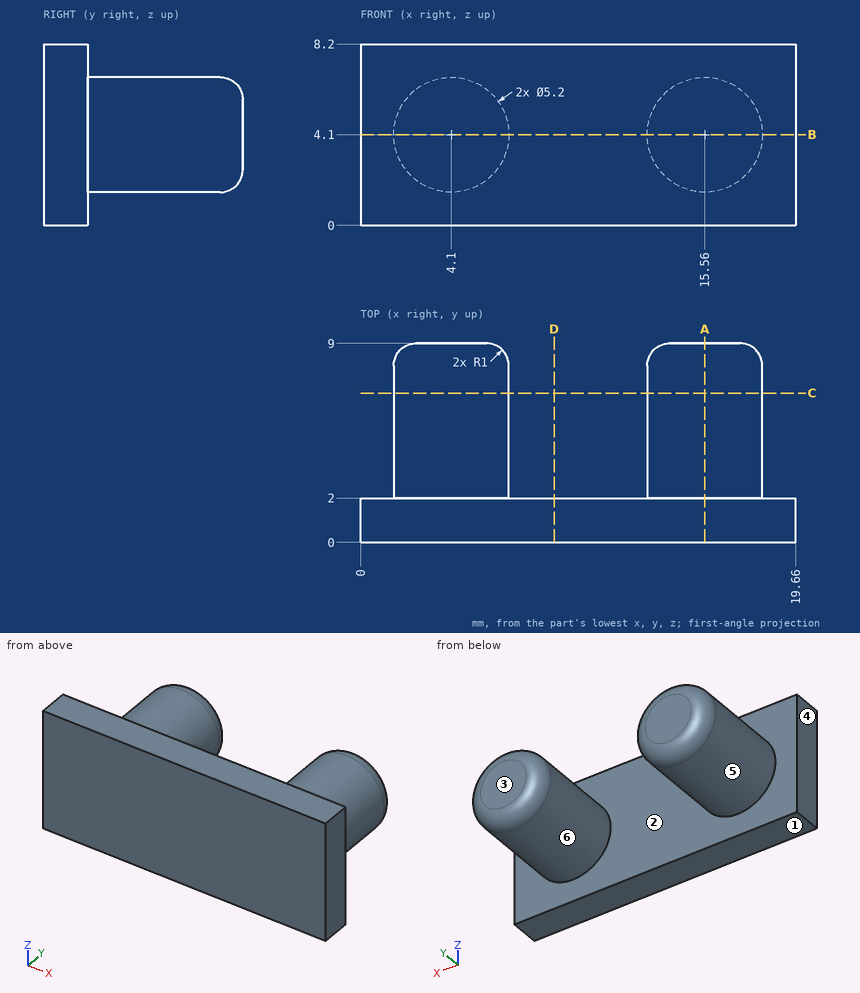
Can you work these out from the drawing? Everything is in mm from the part's minimum corner. A direction names the side the tool comes from. Round coordinates to 2 decimals unless told otherwise and drop trailing zeros. Loops run counter-clockwise (first coordinate to the right, second up) from the corner with the lowest first, then second, coordinate; pieces in that order, holes last. Notation, with made-up numbers: (-36.5, -1.75) -> (-7.5, -1.75) arc R20 cw to (-7.5, 7.25) -> close; hole circle Ø9 at (28, -1). An arc over 180 degrees is marked (long way). Put each result on its own line as item: value.
Q1. I want a section at B-B on z = 4.1. Write out the boundary of the cut face in (x, y), and give its area (3 significant figures).
Checks:
outline: (0, 0) -> (19.66, 0) -> (19.66, 2) -> (18.16, 2) -> (18.16, 8) arc R1 ccw to (17.16, 9) -> (13.96, 9) arc R1 ccw to (12.96, 8) -> (12.96, 2) -> (6.7, 2) -> (6.7, 8) arc R1 ccw to (5.7, 9) -> (2.5, 9) arc R1 ccw to (1.5, 8) -> (1.5, 2) -> (0, 2) -> close
area: 111 mm2
Q2. I want a section at A-A on x = 15.56. Write out the boundary of the cut face in (y, z).
Checks:
outline: (0, 0) -> (2, 0) -> (2, 1.5) -> (8, 1.5) arc R1 ccw to (9, 2.5) -> (9, 5.7) arc R1 ccw to (8, 6.7) -> (2, 6.7) -> (2, 8.2) -> (0, 8.2) -> close
Q3. For pin 1 Ø4 at (x, z) = (12.5, 5.5) entering from +Y; pin 2 Ø1 at (x, y) = (11.5, 3.5) entering from -Z, each with a flat end and sliding along its axis, tell me the tip position at first contact or that it passes through.
Checks:
pin 1: y = 9
pin 2: through
Q4. Thinking about a two-plate mould opening in X: for the marked faces 3, 4, 5 and 6, which applies, pulls with the +X half, pulls with the -X half, needs draft (parallel to the pull), parting line crosses it, or undercut?
Checks:
face 3: needs draft
face 4: pulls with the -X half
face 5: undercut
face 6: undercut
Q5. I want a section at C-C on y = 6.75. Write out the boundary of the cut face in (x, z), and give its area (3 significant figures).
Checks:
outline: circle Ø5.2 at (4.1, 4.1); circle Ø5.2 at (15.56, 4.1)
area: 42.5 mm2
Q6. Which directions (+Z, -Z, +X, -X, +Y, -Y) give clear straight access to the entire face, cutting with the end or side of a thin tool? Please do the marked faces 1 and 2.
Checks:
face 1: -Z, +X, -X, +Y, -Y
face 2: +Y
Q7. I want a section at D-D on x = 8.75. Write out the boundary of the cut face in (y, z).
Checks:
outline: (0, 0) -> (2, 0) -> (2, 8.2) -> (0, 8.2) -> close
Q8. Please list where these lines run through material, in increasing order: line 1 (X direction, y = 2.75, z = 4); line 2 (X direction, y = 8.75, z = 3.25); line 3 (Y direction, x = 12.25, z = 1.5). Write a range as from..to.
Checks:
line 1: 1.5..6.7, 12.96..18.16
line 2: 2..6.2, 13.46..17.66
line 3: 0..2
